Geometry: final body of the model. Coordinates: model frame, mm. Give positions to 0.01 mm unless a question says otherwise; leave off trailing zeros. Loops run counter-clockwise (first coordinate to the right, second up) from the corner with the lowest first, then second, coordinate; pieces in that order, holes last. Notation, with made-up numbers: (33, 82) - (77, 82) arc R21 cw to (77, 107) - close; hole circle Ø11 at (4, -18). An arc over 180 degrees is marked (long way). Use one line per item in the form item = value.
```python
from build123d import *

# Parameters (mm, degrees)
RESSALTO_EXTRUS_O1_DEPTH = 2.5


with BuildPart() as part:
    # Esboço1 → Ressalto-extrusão1 (new body)
    with BuildSketch(Plane.YZ):
        with BuildLine():
            ThreePointArc((350.755952356, -100), (377.550871599, 0), (350.755952356, 100))
            ThreePointArc((350.755952356, 100), (340.510761827, 102.745190528), (337.765571299, 92.5))
            ThreePointArc((337.765571299, 92.5), (348.462298659, 70.811609925), (356.238644162, 47.913254287))
            add(Edge.make_bspline(
                [(356.238644162, 47.913254287), (360.34603799, 30.905478266), (357.108936786, 22.632743478), (348.864388441, 5.278932836), (348.785718872, 0)],
                knots=[0.097242939, 0.097242939, 0.097242939, 0.097242939, 0.646678025, 1, 1, 1, 1], degree=3))
            add(Edge.make_bspline(
                [(356.238644162, -47.913254287), (360.34603799, -30.905478266), (357.108936786, -22.632743478), (348.864388441, -5.278932836), (348.785718872, 0)],
                knots=[0.097242939, 0.097242939, 0.097242939, 0.097242939, 0.646678025, 1, 1, 1, 1], degree=3))
            ThreePointArc((356.238644162, -47.913254287), (348.462298659, -70.811609925), (337.765571299, -92.5))
            ThreePointArc((337.765571299, -92.5), (340.510761827, -102.745190528), (350.755952356, -100))
        make_face()
    extrude(amount=RESSALTO_EXTRUS_O1_DEPTH)


solid = part.part
```
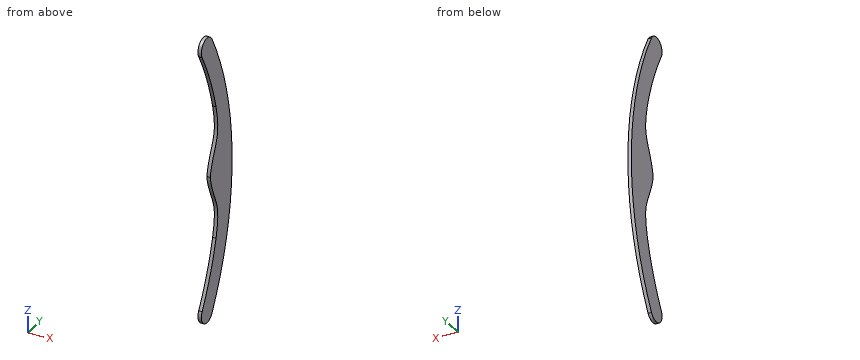
(1) Cut plane C-C (y = 361.5). Return the cut outline in (x, z).
Solution:
outline = (0, -78.5) - (2.5, -78.5) - (2.5, 78.5) - (0, 78.5) - close
(2) Pin query (flat end, axial travel): P1, Ø5, axis at y = 364.5, z = 31, coming from the -X side. Return the tip coordinate at first contact, or that it passes through.
Solution:
P1 = 0
(3) Cut plane A-A (y = 341.5). Return the cut outline in (x, z).
Solution:
outline = (0, -103.22) - (2.5, -103.22) - (2.5, -85.71) - (0, -85.71) - close; (0, 85.71) - (2.5, 85.71) - (2.5, 103.22) - (0, 103.22) - close
(4) Material intervals for L1, parallel to Y at x = 1.8, z = -68.5; L2, parallel to Y at x = 0.9, z = 43; L3, parallel to Z at x = 1.45, y = 359.5, sorted ascending. Write a range as from..to.
Solution:
L1 = 349.4..365.45
L2 = 357.32..372.87
L3 = -83.03..83.03
(5) Cut plane B-B (z = 96.25). Return the cut outline in (x, y), plus the area to 3 significant figures.
Solution:
outline = (0, 336.76) - (2.5, 336.76) - (2.5, 352.87) - (0, 352.87) - close
area = 40.3 mm2
